```python
from build123d import *

# Parameters (mm, degrees)
F0_W     = 420
F0_H     = 75
F1_DEPTH = 270
F2_W     = 400
F2_H     = 250
F3_DEPTH = 65
F5_DEPTH = 420.001


with BuildPart() as f1:
    # F0 (on Front) → F1 (new body)
    with BuildSketch(Plane.XZ):
        with Locations((210, 37.5)):
            Rectangle(F0_W, F0_H)
    extrude(amount=-F1_DEPTH)

    # F2 (on face) → F3 (cut)
    with BuildSketch(Plane.XY.offset(75)):
        with Locations((210, 135)):
            Rectangle(F2_W, F2_H)
    extrude(amount=-F3_DEPTH, mode=Mode.SUBTRACT)

    # F4 (on face) → F5 (cut, through all)
    with BuildSketch(Plane.YZ.offset(420)):
        with BuildLine():
            Line((175, 51), (95, 51))
            ThreePointArc((95, 51), (84, 40), (95, 29))
            Line((95, 29), (175, 29))
            ThreePointArc((175, 29), (186, 40), (175, 51))
        make_face()
    extrude(amount=-F5_DEPTH, mode=Mode.SUBTRACT)


solid = f1.part
```
Here's how the part is built. I have some questions about the finished solid (model axes, mm). A direction names the side the tool comes from. Coordinates: 2 decimals unless noted, no trailing zeros. Write each loop counter-clockwise with the first axis right and the second up, starting at its lowest first coordinate (ties: lowest second). Pieces come first, ordered by that corner, then holes. Notation, with made-up numbers: (7.5, 88) - (23.5, 88) arc R29 cw to (23.5, 112) - close; hole circle Ø5 at (-24.5, 53.25). An arc over 180 degrees is marked (long way). One line per item, written item: value.
1) We'd pull the mould along X, two halves only. Please class faces 4 (the flat face through (207, 133, 0)), 5 (the flat face through (410, 133, 57)), 6 (the flat face through (420, 133.1, 28.6)): pulls with the +X half, pulls with the -X half, needs draft (parallel to the pull), parting line crosses it, or undercut.
Model answer:
face 4: needs draft
face 5: undercut
face 6: pulls with the +X half
2) Suppose I cut it at B-B on y = 126.5. Write out the boundary of the cut face in (x, z), and give its area (3 significant figures).
Model answer:
outline: (0, 0) - (420, 0) - (420, 29) - (410, 29) - (410, 10) - (10, 10) - (10, 29) - (0, 29) - close; (0, 51) - (10, 51) - (10, 75) - (0, 75) - close; (410, 51) - (420, 51) - (420, 75) - (410, 75) - close
area: 5,060 mm²
3) Suppose I cut it at C-C on x = 38.5. Write out the boundary of the cut face in (y, z).
Model answer:
outline: (0, 0) - (270, 0) - (270, 75) - (260, 75) - (260, 10) - (10, 10) - (10, 75) - (0, 75) - close
4) On a 3-axis mill with a long thin cutter (end or side, diameter ignored), from which of +Z, -Z, +X, -X, +Y, -Y can I reach the whole of each face in a straight line? I mean faces 1 (the flat face through (193, 264, 75)), 2 (the flat face through (207, 10, 43)), 3 (the cylindrical face through (415, 186, 40)). Say none if no direction works.
Model answer:
face 1: +Z, +X, -X, +Y, -Y
face 2: +Z
face 3: +X, -X
5) Suppose I cut it at A-A on z = 40. Write out the boundary of the cut face in (x, y), and give its area (3 significant figures).
Model answer:
outline: (0, 0) - (420, 0) - (420, 84) - (410, 84) - (410, 10) - (10, 10) - (10, 84) - (0, 84) - close; (0, 186) - (10, 186) - (10, 260) - (410, 260) - (410, 186) - (420, 186) - (420, 270) - (0, 270) - close
area: 11,400 mm²
6) Suppose I cut it at D-D on y = 18.5. Write out the boundary of the cut face in (x, z).
Model answer:
outline: (0, 0) - (420, 0) - (420, 75) - (410, 75) - (410, 10) - (10, 10) - (10, 75) - (0, 75) - close
7) I need wall thicknesses on line 1 along Y through (x, z) = (377.5, 53); line 2 along X through (y, z) = (237, 64); line 3 along Z through (x, y) = (203, 169). Which ranges of each line are inside material? Lowest first, please.
Model answer:
line 1: y = 0 to 10, 260 to 270
line 2: x = 0 to 10, 410 to 420
line 3: z = 0 to 10
